Build history of the part. All positions in model axes, mm. A direction names the side the tool comes from. Round coordinates to 2 decimals unless told otherwise and drop trailing zeros. Loops run counter-clockwise (first coordinate to the right, second up) from the corner with the lowest first, then second, coordinate; pieces in that order, holes last. Notation, with made-up numbers: (40, 30.25) - (68, 30.25) arc R8 ccw to (68, 34.25) - close; hole circle Ø11 at (5, 72.25). An arc over 180 degrees is marked (long way). Use one line per item in the form item = value. Start each with the question number.
Q1. Pin check, flat tips, straight feed: pin 1 (0.9 mm diameter, centred on x = 5.5, z = 2.5, fed in from +Y); pin 2 (1.2 mm diameter, centred on x = -9, z = 7, fed in from -Y); pin 3 (3.5 mm diameter, centred on x = 3, z = 2, fed in from -Y). Stop position of each tip, or through.
Q2. Saw through at A-A (z = 2.5). Give the cut face in (x, y).
Q3. Saw through at C-C (x = -8.5). Give the cut face in (y, z), then the cut area to 3 significant figures.
Q4. Drill centre lines: line 1 (Y direction, x = -8.5, z = 6.75); line 2 (Z direction, x = 6, y = 56.5); line 3 (X direction, y = 2, z = 0.25). Where is each one in solid material? Low to high.
Q5. 3-axis set-ups, long thin cutter, end or side, ignore diameter. For faces 4 (the face through (5, 18, 2)), 5 (the face through (5, 9, 5)), 6 (the face through (-8, 61, 7)), 7 (the face through (-14, 64, 7)), 8 (the face through (5, 5, -2)): which of +Z, -Z, +X, -X, +Y, -Y reach the whole face in a straight line?
Q6. Mould opens along Y. For faces 1 (the face through (-14, 76, 7)), 2 (the face through (-12, 72, 7)), 3 (the face through (5, -2, 7)) say: released by +Y, released by -Y, zero draft, split by the parting line, or undercut.
Q7. Saw through at B-B (y = 9). Give the cut face in (x, z), then the cut area to 3 significant figures.
Q8. Saw through at D-D (z = 11.75). Give the cut face in (x, y).
Autodesk Fusion 360 part; units mm, degrees
sketch "Sketch1" plane through (0, 0, 0) normal (1, 0, 0) x (0, 1, 0)
  line L0 (0, 0) -> (0, 5) construction
  line L1 (0, 5) -> (3, 5) construction
  line L2 (3, 5) -> (3, 0) construction
  line L3 (3, 0) -> (0, 0) construction
  line L4 (0, 5) -> (-2, 5) construction
  line L5 (-2, 5) -> (-2, 9) construction
  line L6 (0, 0) -> (-2, 0) construction
  line L7 (-2, 0) -> (-2, -3) construction
  line L8 (-2, -3) -> (5, -3) construction
  line L9 (5, -3) -> (5, 0) construction
  line L10 (5, 0) -> (3, 0) construction
  line L11 (3, 5) -> (5, 5) construction
  line L12 (5, 5) -> (5, 9) construction
  line L13 (-2, 9) -> (5, 9) construction
  line L14 (-2, 5) -> (0, 5)
  line L15 (0, 5) -> (0, 0)
  line L16 (0, 0) -> (-2, 0)
  line L17 (-2, 0) -> (-2, -3)
  line L18 (-2, -3) -> (5, -3)
  line L19 (5, -3) -> (5, 0)
  line L20 (5, 0) -> (3, 0)
  line L21 (3, 0) -> (3, 5)
  line L22 (3, 5) -> (5, 5)
  line L23 (5, 5) -> (5, 9)
  line L24 (5, 9) -> (-2, 9)
  line L25 (-2, 9) -> (-2, 5)
  line L26 (-2, 5) -> (0, 5)
  line L27 (5, 9) -> (-2, 9)
  line L28 (-2, 0) -> (-2, -3)
  line L29 (3, 5) -> (5, 5) construction
  line L30 (5, 5) -> (5, 9) construction
  line L31 (5, 0) -> (3, 0)
  line L32 (-2, 0) -> (-2, -3) construction
  line L33 (5, 0) -> (3, 0) construction
  line L34 (-2, 9) -> (5, 9) construction
  line L35 (-2, -3) -> (5, -3) construction
  line L36 (-2, -3) -> (5, -3)
  line L37 (-2, 9) -> (-2, 5)
  line L38 (5, -3) -> (5, 0) construction
  line L39 (3, 5) -> (3, 0) construction
  line L40 (5, -3) -> (5, 0)
  line L41 (0, 0) -> (-2, 0)
  line L42 (3, 0) -> (3, 5)
  line L43 (0, 0) -> (-2, 0) construction
  line L44 (-2, 5) -> (-2, 9) construction
  line L45 (0, 5) -> (3, 5) construction
  line L46 (3, 5) -> (5, 5)
  line L47 (5, 5) -> (5, 9)
  line L48 (0, 0) -> (0, 5) construction
  line L49 (3, 0) -> (0, 0) construction
  line L50 (0, 5) -> (-2, 5) construction
  line L51 (0, 5) -> (0, 0)
  line L52 (13, 5) -> (15, 5)
  line L53 (20, 9) -> (13, 9)
  line L54 (13, 0) -> (13, -3)
  line L55 (18, 5) -> (20, 5) construction
  line L56 (20, 5) -> (20, 9) construction
  line L57 (20, 0) -> (18, 0)
  line L58 (13, 0) -> (13, -3) construction
  line L59 (20, 0) -> (18, 0) construction
  line L60 (13, 9) -> (20, 9) construction
  line L61 (13, -3) -> (20, -3) construction
  line L62 (13, -3) -> (20, -3)
  line L63 (13, 9) -> (13, 5)
  line L64 (20, -3) -> (20, 0) construction
  line L65 (18, 5) -> (18, 0) construction
  line L66 (20, -3) -> (20, 0)
  line L67 (15, 0) -> (13, 0)
  line L68 (18, 0) -> (18, 5)
  line L69 (15, 0) -> (13, 0) construction
  line L70 (13, 5) -> (13, 9) construction
  line L71 (15, 5) -> (18, 5) construction
  line L72 (18, 5) -> (20, 5)
  line L73 (20, 5) -> (20, 9)
  line L74 (15, 0) -> (15, 5) construction
  line L75 (18, 0) -> (15, 0) construction
  line L76 (15, 5) -> (13, 5) construction
  line L77 (15, 5) -> (15, 0)
  point P0 (15, 0)
  dimension "d1" = 5
  dimension "d2" = 3
  dimension "d3" = 2
  dimension "d4" = 4
  dimension "d5" = 3
  dimension "d6" = 2
  dimension "d7" = 4
  dimension "d8" = 5
  dimension "d9" = 3
  dimension "d10" = 2
  dimension "d11" = 4
  dimension "d12" = 3
  dimension "d13" = 2
  dimension "d14" = 4
  dimension "d15" = 5
  dimension "d16" = 3
  dimension "d17" = 2
  dimension "d18" = 4
  dimension "d19" = 3
  dimension "d20" = 2
  dimension "d21" = 4
extrude "Extrude1" add sketch "Sketch1" along normal blind 10 makes body 1 at (6.6667, 0.3333, -3) makes body 2 at (3.3333, 15.3333, -3)
extrude "Extrude2" add 1 faces at (3.3333, 5, 6.3333) along direction (0, 1, 0) blind 8 on bodies 1 bodies 1 2
fillet "Fillet1" radius 1 1 edges at (5, 18, 5) on bodies 1
fillet "Fillet2" radius 1 1 edges at (5, 18, 0) on bodies 1
fillet "Fillet3" radius 1 1 edges at (5, 15, 0) on bodies 1
fillet "Fillet4" radius 1 1 edges at (5, 15, 5) on bodies 1
fillet "Fillet5" radius 1 1 edges at (5, 3, 0) on bodies 1
fillet "Fillet6" radius 1 1 edges at (5, 0, 0) on bodies 1
fillet "Fillet7" radius 1 1 edges at (5, 0, 5) on bodies 1
fillet "Fillet8" radius 1 1 edges at (5, 3, 5) on bodies 1
extrude "Extrude3" add 1 faces at (3.3333, 20, 6.3333) along direction (0, 1, 0) blind 59 on bodies 1 bodies 1
sketch "Sketch2" plane through (0, 0, 9) normal (0, 0, 1) x (-1, 0, 0)
  line L0 (0, -5) -> (-10, -5)
  line L1 (-10, -5) -> (-10, -13)
  line L2 (-10, -13) -> (0, -13)
  line L3 (0, -13) -> (0, -5)
  line L4 (-5, -13) -> (-5, -9) construction
  circle A0 centre (-5, -9) radius 2.5
  dimension "d44" = 5
extrude "Extrude4" add sketch "Sketch2" along normal blind 5 contours A0 bodies 1
sketch "Sketch3" plane through (0, 0, 0) normal (-1, 0, 0) x (0, -1, 0)
  arc A0 (1, 5) -> (0, 4) centre (1, 4) ccw
  line L0 (1, 5) -> (2, 5)
  line L1 (2, 5) -> (2, 9)
  line L2 (2, 9) -> (-5, 9)
  line L3 (-5, 9) -> (-13, 9)
  line L4 (-13, 9) -> (-20, 9)
  line L5 (-20, 9) -> (-79, 9)
  line L6 (-79, 9) -> (-79, 5)
  line L7 (-79, 5) -> (-19, 5)
  arc A1 (-18, 4) -> (-19, 5) centre (-19, 4) ccw
  line L8 (-18, 4) -> (-18, 1)
  arc A2 (-19, 0) -> (-18, 1) centre (-19, 1) ccw
  line L9 (-19, 0) -> (-20, 0)
  line L10 (-20, 0) -> (-20, -3)
  line L11 (-20, -3) -> (-13, -3)
  line L12 (-13, -3) -> (-13, 0)
  line L13 (-13, 0) -> (-14, 0)
  arc A3 (-15, 1) -> (-14, 0) centre (-14, 1) ccw
  line L14 (-15, 1) -> (-15, 4)
  arc A4 (-14, 5) -> (-15, 4) centre (-14, 4) ccw
  line L15 (-14, 5) -> (-4, 5)
  arc A5 (-3, 4) -> (-4, 5) centre (-4, 4) ccw
  line L16 (-3, 4) -> (-3, 1)
  arc A6 (-4, 0) -> (-3, 1) centre (-4, 1) ccw
  line L17 (-4, 0) -> (-5, 0)
  line L18 (-5, 0) -> (-5, -3)
  line L19 (-5, -3) -> (2, -3)
  line L20 (2, -3) -> (2, 0)
  line L21 (2, 0) -> (1, 0)
  arc A7 (0, 1) -> (1, 0) centre (1, 1) ccw
  line L22 (0, 1) -> (0, 4)
  line L23 (-79, 9) -> (-61, 9)
  line L24 (-61, 9) -> (-61, 5)
  line L25 (-61, 5) -> (-79, 5)
  line L26 (-79, 5) -> (-79, 9)
  dimension "d47" = 18
extrude "Extrude5" add sketch "Sketch3" along normal blind 14 contours L5 L6 L7 L23 L24 L25 L26 bodies 1
fillet "Fillet9" radius 5 1 edges at (0, 61, 7) on bodies 1
fillet "Fillet10" radius 5 1 edges at (10, 79, 7) on bodies 1
sketch "Sketch4" plane through (0, 0, 9) normal (0, 0, 1) x (-1, 0, 0)
  arc A0 (-10, -74) -> (-5, -79) centre (-5, -74) ccw
  line L0 (-5, -79) -> (14, -79)
  line L1 (14, -79) -> (14, -61)
  line L2 (14, -61) -> (5, -61)
  arc A1 (0, -56) -> (5, -61) centre (5, -56) ccw
  line L3 (0, -56) -> (0, -20)
  line L4 (0, -20) -> (-10, -20)
  line L5 (-10, -20) -> (-10, -74)
  line L6 (16, -79) -> (12, -79) construction
  line L7 (12, -79) -> (12, -61) construction
  line L8 (12, -61) -> (16, -61) construction
  line L9 (16, -61) -> (16, -79) construction
  line L10 (12, -79) -> (12, -77) construction
  line L11 (12, -77) -> (16, -76) construction
  line L12 (16, -76) -> (16, -74) construction
  line L13 (16, -74) -> (12, -73) construction
  line L14 (12, -71) -> (16, -70) construction
  line L15 (16, -70) -> (16, -68) construction
  line L16 (16, -68) -> (12, -67) construction
  line L17 (12, -65) -> (16, -64) construction
  line L18 (16, -62) -> (12, -61) construction
  line L19 (12, -76.5) -> (16, -75.5) construction
  line L20 (16, -74.5) -> (12, -73.5) construction
  line L21 (16, -68.5) -> (12, -67.5) construction
  line L22 (16, -69.5) -> (12, -70.5) construction
  line L23 (16, -62.5) -> (12, -61.5) construction
  line L24 (16, -63.5) -> (12, -64.5) construction
  line L25 (15.4977, -62.3744) -> (15.4977, -63.6256)
  line L26 (15.4977, -68.3744) -> (15.4977, -69.6256)
  line L27 (15.4787, -74.3697) -> (15.4787, -75.6303)
  line L28 (15.4787, -75.6303) -> (12, -76.5)
  line L29 (15.4787, -74.3697) -> (12, -73.5)
  line L30 (15.4977, -69.6256) -> (12, -70.5)
  line L31 (15.4977, -68.3744) -> (12, -67.5)
  line L32 (15.4977, -63.6256) -> (12, -64.5)
  line L33 (15.4977, -62.3744) -> (12, -61.5)
  line L34 (13.925, -70.0187) -> (14, -74)
  line L35 (14, -76) -> (14, -79)
  line L36 (14, -62) -> (14, -61)
  line L37 (12, -61) -> (12, -61.5)
  line L38 (12, -64.5) -> (12, -67.5)
  line L39 (14, -64) -> (14, -68)
  line L40 (12, -70.5) -> (12, -73.5)
  line L41 (12, -76.5) -> (12, -79)
  line L42 (14, -79) -> (12, -79)
extrude "Extrude6" add sketch "Sketch4" against normal blind 4 contours L1 L27 L28 L29 | L1 L26 L30 L31 | L1 L25 L32 L33 bodies 1
extrude "Extrude7" cut sketch "Sketch4" against normal blind 4 contours L0 L1 L28 L35 L41 L42 | L29 L30 L34 L40 | L1 L2 L33 L36 L37 | L1 L31 L32 L38 L39 bodies 1
extrude "Extrude8" cut 1 faces at (-14, 72.6667, 7.6667) along direction (1, 0, 0) blind 0.1 on bodies 1 bodies 1
Report:
q1.pin_1 = 18
q1.pin_2 = 61
q1.pin_3 = -0.34
q2.outline = (0, 0) - (10, 0) - (10, 3) - (0, 3) - close; (0, 15) - (10, 15) - (10, 18) - (0, 18) - close
q3.outline = (61, 5) - (79, 5) - (79, 9) - (61, 9) - close
q3.area = 72.0 mm²
q4.line_1 = 61 to 79
q4.line_2 = 5 to 9
q4.line_3 = 0 to 10
q5.face_4 = +X, -X, +Y
q5.face_5 = +X, -X
q5.face_6 = +Z, -Z, -X, -Y
q5.face_7 = +Z, -Z, -X
q5.face_8 = -Z, +X, -X
q6.face_1 = released by +Y
q6.face_2 = undercut
q6.face_3 = released by -Y
q7.outline = (0, 5) - (10, 5) - (10, 9) - (7.5, 9) - (7.5, 14) - (2.5, 14) - (2.5, 9) - (0, 9) - close
q7.area = 65.0 mm²
q8.outline = circle Ø5 at (5, 9)
